```python
from build123d import *

# Parameters (mm, degrees)
SKETCH_1_R             = 32
EXTRUDE_1_DEPTH        = 5
SKETCH_5_R             = 16
EXTRUDE_2_DEPTH        = 5
SKETCH_7_R             = 32
EXTRUDE_4_DEPTH        = 37.3
CUT_EXTRUDE_1_DEPTH    = 5
SKETCH_11_R            = 3
EXTRUDE_5_DEPTH        = 10
SKETCH_12_R            = 1
CUT_EXTRUDE_3_DEPTH    = 10
HOLE_WIZARD_M3_1_D     = 2.5
HOLE_WIZARD_M3_1_DEPTH = 14.9
HOLE_WIZARD_M3_1_TIP   = 0.751075774


with BuildPart() as part:
    # Sketch 3 → Revolve 1 (revolve)
    with BuildSketch(Plane.XY):
        with BuildLine():
            Line((0, 0), (0, -16))
            add(Edge.make_bspline(
                [(0, -16), (22.5, -8), (25, 0)],
                knots=[0, 0, 0, 1, 1, 1], degree=2))
            Line((25, 0), (0, 0))
        make_face()
    revolve(axis=Axis((25, 0, 0), (-1, 0, 0)))



with BuildPart() as body_2:
    # Sketch 1 → Extrude 1 (new body)
    # profile 1 of 4: a face of its own
    with BuildSketch(Plane(origin=(0, 0, 0), x_dir=(0, 0, -1), z_dir=(1, 0, 0))):
        with BuildLine():
            Line((47, 12), (34.290944869, 12))
            ThreePointArc((34.290944869, 12), (-36.33, 0), (34.290944869, -12))
            Line((34.290944869, -12), (47, -12))
            Line((47, -12), (47, 12))
        make_face()
        Circle(SKETCH_1_R, mode=Mode.SUBTRACT)
    # profile 2 of 4: a face of its own
    with BuildSketch(Plane(origin=(0, 0, 0), x_dir=(0, 0, -1), z_dir=(1, 0, 0))):
        with BuildLine():
            ThreePointArc((-15.803480629, -2.5), (-16, 0), (-15.803480629, 2.5))
            Line((-15.803480629, 2.5), (-31.902194282, 2.5))
            ThreePointArc((-31.902194282, 2.5), (-32, 0), (-31.902194282, -2.5))
            Line((-31.902194282, -2.5), (-15.803480629, -2.5))
        make_face()
    # profile 3 of 4: a face of its own
    with BuildSketch(Plane(origin=(0, 0, 0), x_dir=(0, 0, -1), z_dir=(1, 0, 0))):
        with BuildLine():
            Line((13.786033631, 28.878110685), (5.736676805, 14.936215693))
            ThreePointArc((5.736676805, 14.936215693), (8, 13.856406461), (10.066803824, 12.436215693))
            Line((10.066803824, 12.436215693), (18.11616065, 26.378110685))
            ThreePointArc((18.11616065, 26.378110685), (16, 27.712812921), (13.786033631, 28.878110685))
        make_face()
    # profile 4 of 4: a face of its own
    with BuildSketch(Plane(origin=(0, 0, 0), x_dir=(0, 0, -1), z_dir=(1, 0, 0))):
        with BuildLine():
            Line((18.11616065, -26.378110685), (10.066803824, -12.436215693))
            ThreePointArc((10.066803824, -12.436215693), (8, -13.856406461), (5.736676805, -14.936215693))
            Line((5.736676805, -14.936215693), (13.786033631, -28.878110685))
            ThreePointArc((13.786033631, -28.878110685), (16, -27.712812921), (18.11616065, -26.378110685))
        make_face()
    extrude(amount=-EXTRUDE_1_DEPTH)


with BuildPart() as part_1:
    add(part.part)

    add(body_2.part)  # Extrude 2 merges body 2
    # Sketch 5 → Extrude 2 (add)
    with BuildSketch(Plane.ZY):
        Circle(SKETCH_5_R)
    extrude(amount=EXTRUDE_2_DEPTH)

    # Sketch 7 → Extrude 4 (add)
    with BuildSketch(Plane.ZY.offset(5)):
        with BuildLine():
            Line((-34.290944869, 12), (-47, 12))
            Line((-47, 12), (-47, -12))
            Line((-47, -12), (-34.290944869, -12))
            ThreePointArc((-34.290944869, -12), (36.33, 0), (-34.290944869, 12))
        make_face()
        with Locations(Location((0, 0, 0), (0, 0, 124.480798786))):
            Circle(SKETCH_7_R, mode=Mode.SUBTRACT)
    extrude(amount=EXTRUDE_4_DEPTH)

    # Sketch 9 → Cut-Extrude 1 (cut)
    with BuildSketch(Plane(origin=(0, 0, -47), x_dir=(-1, 0, 0), z_dir=(0, 0, -1))):
        with BuildLine():
            Line((42.3, -4), (42.3, 4))
            ThreePointArc((42.3, 4), (39.699643621, 2.707512696), (38.65, 0))
            ThreePointArc((38.65, 0), (39.699643621, -2.707512696), (42.3, -4))
        make_face()
    extrude(amount=-CUT_EXTRUDE_1_DEPTH, mode=Mode.SUBTRACT)

    # Sketch 11 → Extrude 5 (add)
    with BuildSketch(Plane.ZY.offset(5)):
        Circle(SKETCH_11_R)
    extrude(amount=EXTRUDE_5_DEPTH)

    # Sketch 12 → Cut-Extrude 3 (cut)
    with BuildSketch(Plane.ZY.offset(42.3)):
        with Locations((34, 0)):
            Circle(SKETCH_12_R)
        with Locations((-17, 29.444863729)):
            Circle(SKETCH_12_R)
        with Locations((-17, -29.444863729)):
            Circle(SKETCH_12_R)
    extrude(amount=-CUT_EXTRUDE_3_DEPTH, mode=Mode.SUBTRACT)

    # Hole Wizard M3 _1
    with Locations(Plane(origin=(0, 0, -47), x_dir=(-1, 0, 0), z_dir=(0, 0, -1))):
        with Locations((3.65, -8), (3.65, 8), (38.65, 8), (38.65, -8)):
            Hole(HOLE_WIZARD_M3_1_D / 2, depth=HOLE_WIZARD_M3_1_DEPTH)
            with Locations((0, 0, -(HOLE_WIZARD_M3_1_DEPTH + HOLE_WIZARD_M3_1_TIP / 2))):  # 118° drill point
                Cone(0, HOLE_WIZARD_M3_1_D / 2, HOLE_WIZARD_M3_1_TIP, mode=Mode.SUBTRACT)


solid = part_1.part
```
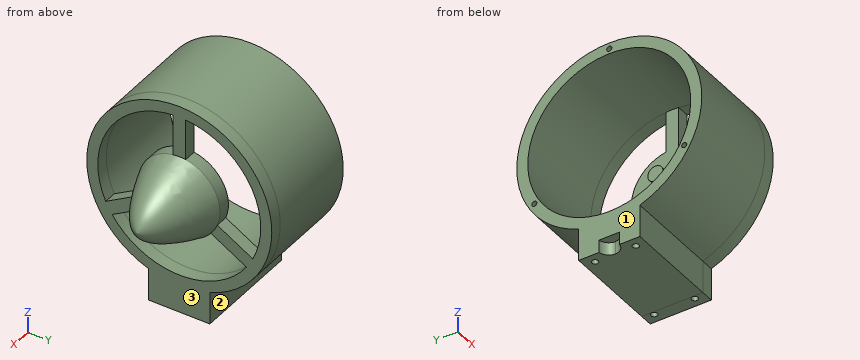
Can you work these out from the model? Positions are in its coordinate system, mm. Face numbers are marked on the shaded views. A direction names the side the tool comes from. Round coordinates to 2 decimals unless told otherwise and drop trailing zeros. Loops run counter-clockwise (first coordinate to the right, second up) from the corner with the lowest first, then second, coordinate; pieces in that order, holes last. Notation, with made-up numbers: M 3,-38 L 22,-38 A7 ccw 22,-26 Z; hole C -25.75,-16.75 d3. An arc over 180 degrees is marked long. Answer as a JSON object with one key per item and string values. Group by question number.
Q1. Imagine slicing it at C-C, the plane y = -22. Please give me the cut outline in (x, z).
Q2. Imagine slicing it at B-B, the plane z = -39.5. Please give me the cut outline in (x, y), then the cut area to 3 significant figures.
Q3. Imagine slicing it at A-A, the plane x = -25. Please give me the cut outline in (y, z).
Q4. Please list where these lines run through material, in increasing order: L1, parallel to Y at x = -38.65, z = -36.5; L2, parallel to X at y = 8, z = -42; L3, parallel to X at y = -8.5, z = -42.
Q5. On a 3-axis mill with a long thin cutter (end or side, diameter ignored), from which of +Z, -Z, +X, -X, +Y, -Y can I reach the whole of each face in a straight line? I mean the marked faces 1, 2 and 3. Say none if no direction works.
Q6. Imagine slicing it at D-D, the plane z = 29. Please give me the cut outline in (x, y), then the cut area to 3 significant figures.
Q7. Will these pins go through, and if not, where does the flat tip stop? pin 1 (6.5 mm diameter, centred on x = -23.5, z = -42, fed in from +Y); pin 2 (1.2 mm diameter, centred on y = 29.44, z = -17, fed in from -X); pin 3 (14 mm diameter, centred on x = -18.5, z = -38, fed in from -Y).
Findings:
{
 "1": {"outline": "M -42.3,-28.91 L 0,-28.91 L 0,-23.24 L -42.3,-23.24 Z; M -42.3,23.24 L 0,23.24 L 0,28.91 L -42.3,28.91 Z; M -5,-15.59 L 0,-15.59 L 0,-9.81 L -5,-9.81 Z"},
 "2": {"outline": "M -42.3,-12 L 0,-12 L 0,12 L -42.3,12 Z; hole C -38.65,-8 d2.5; hole C -38.65,8 d2.5; hole C -3.65,-8 d2.5; hole C -3.65,8 d2.5", "area": "996 mm2"},
 "3": {"outline": "M -12,-47 L 12,-47 L 12,-34.29 A36.33 ccw long -12,-34.29 Z; hole C 0,0 d64"},
 "4": {"L1": "y = -12 to -9.25, -6.75 to 6.75, 9.25 to 12", "L2": "x = -42.3 to -39.9, -37.4 to -4.9, -2.4 to 0", "L3": "x = -42.3 to -39.8, -37.5 to -4.8, -2.5 to 0"},
 "5": {"face 1": "+Z, -Z, -X, +Y, -Y", "face 2": "-Z, +X, -X, +Y", "face 3": "+X"},
 "6": {"outline": "M -42.3,-21.88 L 0,-21.88 L 0,-13.53 L -42.3,-13.53 Z; M -42.3,13.53 L 0,13.53 L 0,21.88 L -42.3,21.88 Z; M -5,-2.5 L 0,-2.5 L 0,2.5 L -5,2.5 Z", "area": "732 mm2"},
 "7": {"pin 1": "stops at y = 12", "pin 2": "stops at x = -32.3", "pin 3": "stops at y = -18.94"}
}
